The listing builds one solid part. Answer for the finished solid, in the listing's coordinates (mm). Face numbers are marked on the shaded views. Coordinates: 2 decimals unless noted, no trailing zeros. Write each loop counter-clockwise with the first axis right and the second up, starting at its lowest first coordinate (ties: lowest second). Pieces come first, ordered by that corner, then holes.
(1) The part is cut by section D-D on z = 31.25. Determine the outline of the cut face in (x, y), plus the area to 3 significant figures.
(2) For a pull along Z with two mould halves and no side action, classify the marked faces 1, 2, 3 and 4 as +Z half, -Z half, draft (parallel to the pull), parting line (faces both ways), or undercut.
(3) Straight lines are drawn through the part: line 1 (X direction, y = 3.75, z = 31.25); line 2 (X direction, y = 8.5, z = -63.5); line 3 (X direction, y = 9, z = -8.5). For each, find the intervals that lie inside material, in ascending order.
(4) The part is cut by section C-C on x = 0. Determine the outline of the cut face in (y, z).
(5) The part is cut by section B-B on y = 8.75. Determine the outline of the cut face in (x, z), plus the area to 3 significant figures.
(6) The part is cut by section A-A on z = -62.5. Determine the outline of the cut face in (x, y).
(7) Given P1, Ø1.5, axis at y = 10, z = 23.5, coming from the +X side; P2, Ø2, axis at x = -52.5, y = 3, coming from the +Z side; P3, Ø1.5, axis at y = 2.5, z = -46, coming from the -X side, each flat-ended and moving along its own axis, determine where each tip first touches the part or whether it passes through.
from build123d import *

# Parameters (mm, degrees)
SKETCH1_R           = 75
BOSS_EXTRUDE1_DEPTH = 14
SKETCH2_R           = 13
CUT_EXTRUDE1_DEPTH  = 8
SKETCH3_R           = 12
CUT_EXTRUDE2_DEPTH  = 8
SKETCH4_R           = 5
CUT_EXTRUDE4_DEPTH  = 107.98598039
SKETCH5_R           = 1.75
CUT_EXTRUDE5_DEPTH  = 107.98598039
CUT_EXTRUDE6_DEPTH  = 15


with BuildPart() as part:
    # Sketch1 → Boss-Extrude1 (new body)
    with BuildSketch(Plane(origin=(0, 0, 0), x_dir=(1, 0, 0), z_dir=(0, 1, 0))):
        with Locations(Location((0, 0, 0), (0, 0, 270))):
            Circle(SKETCH1_R)
    extrude(amount=BOSS_EXTRUDE1_DEPTH)

    # Sketch2 → Cut-Extrude1 (cut)
    with BuildSketch(Plane(origin=(0, 14, 0), x_dir=(1, 0, 0), z_dir=(0, 1, 0))):
        with Locations(Location((0, 0, 0), (0, 0, 270))):
            Circle(SKETCH2_R)
    extrude(amount=-CUT_EXTRUDE1_DEPTH, mode=Mode.SUBTRACT)

    # Sketch3 → Cut-Extrude2 (cut)
    with BuildSketch(Plane(origin=(0, 6, 0), x_dir=(1, 0, 0), z_dir=(0, 1, 0))):
        with Locations(Location((0, 0, 0), (0, 0, 270))):
            Circle(SKETCH3_R)
    extrude(amount=-CUT_EXTRUDE2_DEPTH, mode=Mode.SUBTRACT)

    # Sketch4 → Cut-Extrude4 (cut, through all)
    with BuildSketch(Plane(origin=(0, 14, 0), x_dir=(1, 0, 0), z_dir=(0, 1, 0))):
        with Locations(Location((0, 62.5, 0), (0, 0, 270))):
            Circle(SKETCH4_R)
        with Locations(Location((-54.126587737, -31.25, 0), (0, 0, 270))):
            Circle(SKETCH4_R)
        with Locations(Location((54.126587737, -31.25, 0), (0, 0, 270))):
            Circle(SKETCH4_R)
    extrude(amount=-CUT_EXTRUDE4_DEPTH, mode=Mode.SUBTRACT)

    # Sketch5 → Cut-Extrude5 (cut, through all)
    with BuildSketch(Plane(origin=(0, 14, 0), x_dir=(1, 0, 0), z_dir=(0, 1, 0))):
        with Locations(Location((-15.201634245, -47.250661584, 0), (0, 0, 270))):
            Circle(SKETCH5_R)
        with Locations(Location((10.798365755, -47.250661584, 0), (0, 0, 270))):
            Circle(SKETCH5_R)
    extrude(amount=-CUT_EXTRUDE5_DEPTH, mode=Mode.SUBTRACT)

    # Sketch6 → Cut-Extrude6 (cut)
    with BuildSketch(Plane(origin=(0, 0, 0), x_dir=(-1, 0, 0), z_dir=(0, -1, 0))):
        with BuildLine():
            ThreePointArc((75, 0), (54.10858072, 51.935166241), (3.073026868, 74.937016927))
            Line((3.073026868, 74.937016927), (66.751084117, -34.194923151))
            ThreePointArc((66.751084117, -34.194923151), (72.908611661, -17.587903389), (75, 0))
        make_face()
        with BuildLine():
            Line((-65.762802754, -36.059031794), (-3.073026868, 74.937016927))
            ThreePointArc((-3.073026868, 74.937016927), (-65.304085384, 36.883281201), (-65.762802754, -36.059031794))
        make_face()
        with BuildLine():
            ThreePointArc((-63.846861253, -39.351979723), (0.783642911, -74.995905914), (64.655219699, -38.009243162))
            Line((64.655219699, -38.009243162), (25.54691352, -38.417891428))
            ThreePointArc((25.54691352, -38.417891428), (2.039914544, -56.722875597), (-21.844452804, -38.91309057))
            Line((-21.844452804, -38.91309057), (-63.846861253, -39.351979723))
        make_face()
    extrude(amount=-CUT_EXTRUDE6_DEPTH, mode=Mode.SUBTRACT)


solid = part.part
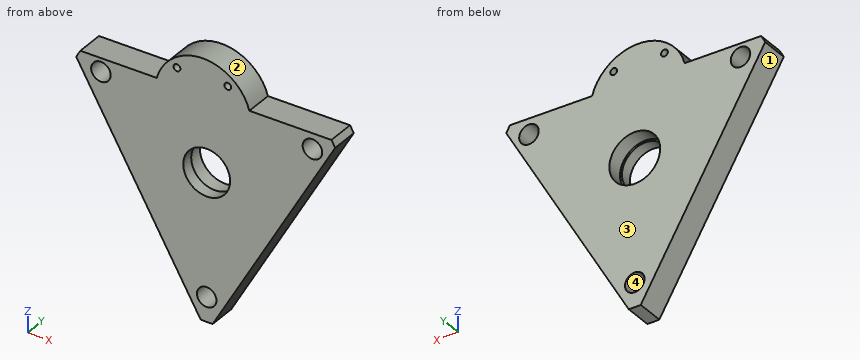
Model answer:
1. outline: (-65.03, 0) - (-59.13, 0) - (-59.13, 14) - (-65.03, 14) - close; (-49.13, 0) - (49.13, 0) - (49.13, 14) - (-49.13, 14) - close; (59.13, 0) - (63.05, 0) - (63.05, 14) - (59.13, 14) - close
1. area: 1,510 mm2
2. face 1: -Z half
2. face 2: +Z half
2. face 3: draft
2. face 4: undercut
3. line 1: x = -65.03 to -59.13, -49.13 to 49.13, 59.13 to 63.05
3. line 2: x = -9.75 to -4.9, 4.9 to 9.53
3. line 3: x = -41.84 to -9.84, 9.84 to 40.6
4. outline: (0, -75) - (14, -75) - (14, -67.5) - (0, -67.5) - close; (0, -57.5) - (14, -57.5) - (14, -13) - (6, -13) - (6, -12) - (0, -12) - close; (0, 12) - (6, 12) - (6, 13) - (14, 13) - (14, 56.66) - (0, 56.66) - close
5. outline: (-66.75, 34.19) - (-3.07, -74.94) arc R75 ccw to (3.07, -74.94) - (65.76, 36.06) arc R75 ccw to (63.85, 39.35) - (21.84, 38.91) arc R24.58 ccw to (-25.55, 38.42) - (-64.66, 38.01) arc R75 ccw to start; hole circle Ø10 at (-54.13, 31.25); hole circle Ø3.5 at (-15.2, 47.25); hole circle Ø26 at (0, 0); hole circle Ø10 at (0, -62.5); hole circle Ø3.5 at (10.8, 47.25); hole circle Ø10 at (54.13, 31.25)
5. area: 7,940 mm2
6. outline: (-10.33, 0) - (-5, 0) - (-5, 14) - (-10.33, 14) - close; (5, 0) - (10.1, 0) - (10.1, 14) - (5, 14) - close
7. P1: stops at x = 59.09
7. P2: stops at z = 38.15
7. P3: stops at x = -20.4
